Here's how the part is built. I have some questions about the finished solid (model axes, mm). A direction names the side the tool comes from. Round coordinates to 2 decimals unless told otherwise and drop trailing zeros. Write each loop counter-clockwise with the first axis right and the second up, starting at its lowest first coordinate (ties: lowest second). Pieces come first, ordered by that corner, then holes. Notation, with made-up numbers: M 37,50 L 70,50 A16 ccw 70,72 Z; hole C 57,21 d6. An arc over 180 degrees is marked long. Use one line per item in the form item = value. Start each with the question number.
Q1. I need wall thicknesses on line 1 along Y through (x, z) = (-916, -33.5); line 2 along Z through (x, y) = (-86.5, -291) (3 decimals); line 3 along X through (y, z) = (-521.5, -20) (3 decimals). Which ranges of each line are inside material? Lowest first, please. Write a range as from..to.
Q2. I want a section at C-C on z = -60.5. List the corners of the cut face in (x, y) for me.
Q3. I'm going to push flat-ended pins straight in: pin 1 Ø6 at (x, z) = (-764, -73.5) entering from -Y; pin 2 Ø16 at (y, z) = (-616.5, -21.5) entering from -X (3 decimals); pin 3 Ø1.6 at (y, z) = (-646.5, -151) entering from +X (3 decimals); pin 4 Ø8 at (y, z) = (-254, -127.5) entering from +X. Where does each tip first touch, or does it pass through?
Q4. I want a section at A-A on x = -953.5. List the corners of the cut face in (y, z) for me (3 decimals).
Q5. For faces 1 (the face through (-304.8, -605, -91)), 2 (the face through (0, -472, -75)), 3 (the face through (-155, -914.4, -91)), 4 (the face through (-1422.4, -150, -91)), 5 (the face through (-320.675, -621, -16)), which set-ups out of +Z, -Z, +X, -X, +Y, -Y let a thin tool reach every point of the face, with its end or its side?
```python
from build123d import *

# Parameters (mm, degrees)
F4_DEPTH = 152.4
F1_DEPTH = 31.75
F3_DEPTH = 3.175


with BuildPart() as f4:
    # F0 (on Top) → F4 (new body)
    with BuildSketch(Plane.XY):
        Polygon((0, 0), (-1422.4, 0), (-1422.4, -304.8), (-304.8, -304.8), (-304.8, -914.4), (0, -914.4), align=None)
    extrude(amount=-F4_DEPTH)

    # F5 (on face) → F1 (join)
    with BuildSketch(Plane.XY):
        Polygon((0, -930.275), (0, 0), (-1438.275, 0), (-1438.275, -320.675), (-320.675, -320.675), (-320.675, -930.275), align=None)
    extrude(amount=-F1_DEPTH)

    # F2 (on face) → F3 (cut)
    with BuildSketch(Plane(origin=(0, 0, -152.4), x_dir=(1, 0, 0), z_dir=(0, 0, -1))):
        Polygon((-288.925, 288.925), (-1406.525, 288.925), (-1406.525, 15.875), (-1406.525, 0), (0, 0), (0, 898.525), (-15.875, 898.525), (-288.925, 898.525), align=None)
    extrude(amount=-F3_DEPTH, mode=Mode.SUBTRACT)


solid = f4.part
```
Reported:
q1.line_1 = -304.8..0
q1.line_2 = -149.225..0
q1.line_3 = -320.675..0
q2.outline = M -1422.4,-304.8 L -304.8,-304.8 L -304.8,-914.4 L 0,-914.4 L 0,0 L -1422.4,0 Z
q3.pin_1 = -304.8
q3.pin_2 = -320.675
q3.pin_3 = -288.925
q3.pin_4 = 0
q4.outline = M -320.675,-31.75 L -304.8,-31.75 L -304.8,-152.4 L -288.925,-152.4 L -288.925,-149.225 L 0,-149.225 L 0,0 L -320.675,0 Z
q5.face_1 = -Z, -X, -Y
q5.face_2 = +Z, -Z, +X, +Y, -Y
q5.face_3 = -Z, +X, -X, -Y
q5.face_4 = -Z, -X, +Y, -Y
q5.face_5 = +Z, -Z, -X, -Y
